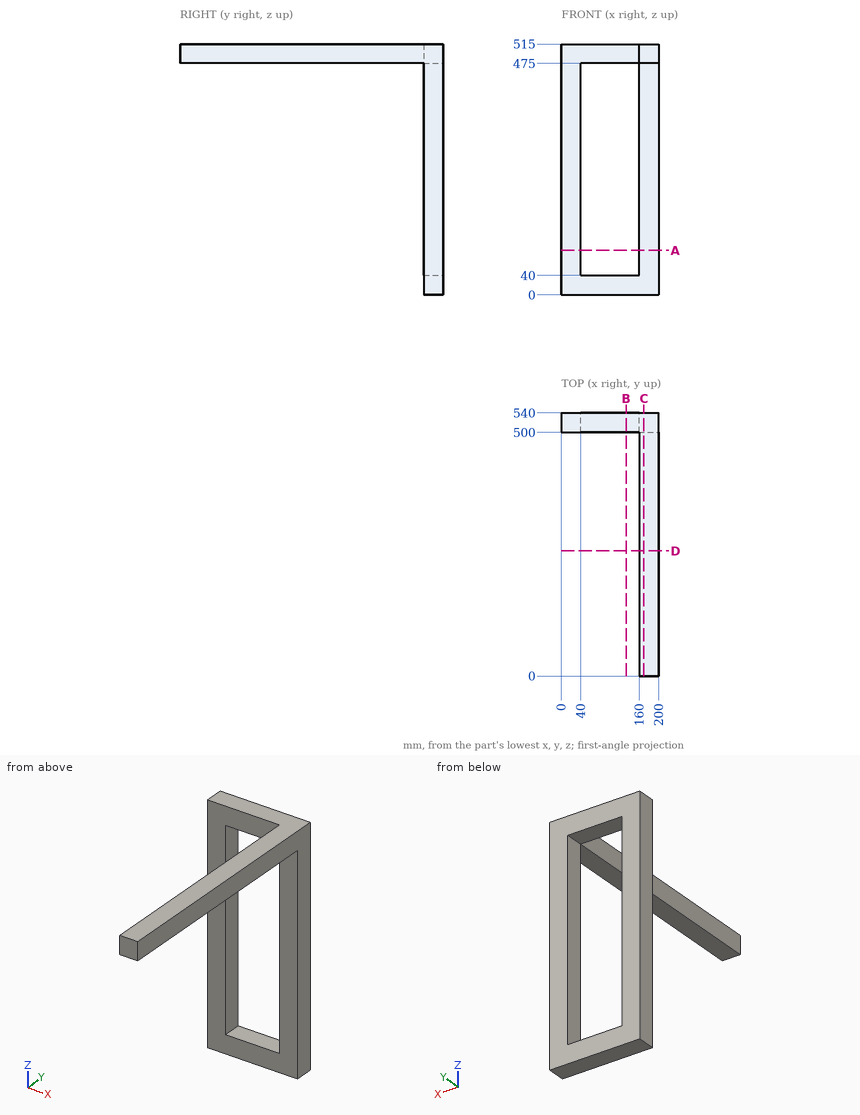
Drawing for the job (mm, zero at the part's lowest x, y, z). Round coordinates to 2 decimals unless told otherwise and drop trailing zeros. Loops run counter-clockwise (first coordinate to the right, second up) from the corner with the lowest first, then second, coordinate; pieces in that order, holes last. Notation, with made-up numbers: (-37.5, -30.5) -> (-13.5, -30.5) arc R21 cw to (-13.5, -9.5) -> close; hole circle Ø11 at (40.5, 0.25). An arc over 180 degrees is marked (long way). Answer as CSV lines item,"result". Start each with the question number.
1) Slice it at A-A (z = 91.5). List the corners of the cut face in (x, y).
2) Pin check, flat tips, straight feed: P1, Ø20, axis at y = 511.5, z = 197, coming from the -X side; P2, Ø20, axis at x = 176.5, y = 166.5, coming from the -Z side. Stop position of each tip, or through.
3) Slice it at B-B (x = 133). List the corners of the cut face in (y, z), plus the area to 3 significant figures.
4) Slice it at D-D (y = 257). List the corners of the cut face in (x, z), plus the area to 3 significant figures.
5) Slice it at C-C (x = 169.5). List the corners of the cut face in (y, z).
6) Probe line 1 along Z through (x, y) = (188, 433); line 2 along Y through (x, z) = (180.5, 330). List the from-to ranges inside material, lowest first.
Filled in:
1,outline,"(0, 500) -> (40, 500) -> (40, 540) -> (0, 540) -> close; (160, 500) -> (200, 500) -> (200, 540) -> (160, 540) -> close"
2,P1,"stops at x = 0"
2,P2,"stops at z = 475"
3,outline,"(500, 0) -> (540, 0) -> (540, 40) -> (500, 40) -> close; (500, 475) -> (540, 475) -> (540, 515) -> (500, 515) -> close"
3,area,"3,200 mm2"
4,outline,"(160, 475) -> (200, 475) -> (200, 515) -> (160, 515) -> close"
4,area,"1,600 mm2"
5,outline,"(0, 475) -> (500, 475) -> (500, 0) -> (540, 0) -> (540, 515) -> (0, 515) -> close"
6,line 1,"z = 475 to 515"
6,line 2,"y = 500 to 540"
